from build123d import *

# Parameters (mm, degrees)
F0_W          = 40.64
F0_H          = 3.81
F1_DEPTH      = 12.7
F2_DEPTH      = 12.6492
F2_DEPTH_BACK = 12.7
F3_D          = 2.54
F3_DEPTH      = 12.701
F4_D          = 2.54
F6_DEPTH      = 4.2291
F7_DEPTH      = 4.2291
F8_D          = 3.81


with BuildPart() as f1:
    # F0 (on Front) → F1 (new body, symmetric)
    with BuildSketch(Plane.XZ):
        Rectangle(F0_W, F0_H)
    extrude(amount=F1_DEPTH, both=True)

    # F0 (on Front) → F2 (join, two sides)
    with BuildSketch(Plane.XZ) as f2_sk:
        with BuildLine():
            Line((20.32, 1.905), (20.32, -1.905))
            Line((20.32, -1.905), (29.8843930952, -0.4539235519))
            ThreePointArc((29.8843930952, -0.4539235519), (29.1094185103, 1.3335), (29.3193590481, 3.2703514481))
            Line((29.3193590481, 3.2703514481), (20.32, 1.905))
        make_face()
        with BuildLine():
            Line((32.8763121576, 0), (29.8843930952, -0.4539235519))
            ThreePointArc((29.8843930952, -0.4539235519), (34.1246887779, -1.6946744039), (36.6863121576, 1.905))
            ThreePointArc((36.6863121576, 1.905), (33.5706134801, 5.6512041687), (29.3193590481, 3.2703514481))
            Line((29.3193590481, 3.2703514481), (32.8763121576, 3.81))
            Line((32.8763121576, 3.81), (32.8763121576, 0))
        make_face()
        with BuildLine():
            ThreePointArc((29.3193590481, 3.2703514481), (29.1094185103, 1.3335), (29.8843930952, -0.4539235519))
            Line((29.8843930952, -0.4539235519), (32.8763121576, 0))
            Line((32.8763121576, 0), (32.8763121576, 3.81))
            Line((32.8763121576, 3.81), (29.3193590481, 3.2703514481))
        make_face()
        with BuildLine():
            Line((-29.8843930952, -0.4539235519), (-20.32, -1.905))
            Line((-20.32, -1.905), (-20.32, 1.905))
            Line((-20.32, 1.905), (-29.3193590481, 3.2703514481))
            ThreePointArc((-29.3193590481, 3.2703514481), (-29.1301079889, 2.5993013225), (-29.0663121576, 1.905))
            ThreePointArc((-29.0663121576, 1.905), (-29.2766377538, 0.6566233797), (-29.8843930952, -0.4539235519))
        make_face()
        with BuildLine():
            ThreePointArc((-29.3193590481, 3.2703514481), (-36.6432058049, 2.4765), (-29.8843930952, -0.4539235519))
            Line((-29.8843930952, -0.4539235519), (-32.8763121576, 0))
            Line((-32.8763121576, 0), (-32.8763121576, 3.81))
            Line((-32.8763121576, 3.81), (-29.3193590481, 3.2703514481))
        make_face()
        with BuildLine():
            Line((-32.8763121576, 0), (-29.8843930952, -0.4539235519))
            ThreePointArc((-29.8843930952, -0.4539235519), (-29.2766377538, 0.6566233797), (-29.0663121576, 1.905))
            ThreePointArc((-29.0663121576, 1.905), (-29.1301079889, 2.5993013225), (-29.3193590481, 3.2703514481))
            Line((-29.3193590481, 3.2703514481), (-32.8763121576, 3.81))
            Line((-32.8763121576, 3.81), (-32.8763121576, 0))
        make_face()
    extrude(amount=F2_DEPTH)
    extrude(f2_sk.sketch, amount=-F2_DEPTH_BACK)

    # F3 (through all, one way)
    with BuildSketch(Plane.XZ):
        with Locations((32.8763121576, 1.905), (-32.8763121576, 1.905)):
            Circle(F3_D / 2)
    extrude(amount=-F3_DEPTH, mode=Mode.SUBTRACT)

    # F4 (through all)
    with Locations(Plane(origin=(0, 0, 0), x_dir=(1, 0, 0), z_dir=(0, 1, 0))):
        with Locations((32.8763121576, -1.905), (-32.8763121576, -1.905)):
            Hole(F4_D / 2)

    # F0 (on Front) → F6 (cut, symmetric)
    with BuildSketch(Plane.XZ):
        with BuildLine():
            Line((20.32, 1.905), (20.32, -1.905))
            Line((20.32, -1.905), (29.8843930952, -0.4539235519))
            ThreePointArc((29.8843930952, -0.4539235519), (29.1094185103, 1.3335), (29.3193590481, 3.2703514481))
            Line((29.3193590481, 3.2703514481), (20.32, 1.905))
        make_face()
        with BuildLine():
            Line((32.8763121576, 0), (29.8843930952, -0.4539235519))
            ThreePointArc((29.8843930952, -0.4539235519), (34.1246887779, -1.6946744039), (36.6863121576, 1.905))
            ThreePointArc((36.6863121576, 1.905), (33.5706134801, 5.6512041687), (29.3193590481, 3.2703514481))
            Line((29.3193590481, 3.2703514481), (32.8763121576, 3.81))
            Line((32.8763121576, 3.81), (32.8763121576, 0))
        make_face()
        with BuildLine():
            ThreePointArc((29.3193590481, 3.2703514481), (29.1094185103, 1.3335), (29.8843930952, -0.4539235519))
            Line((29.8843930952, -0.4539235519), (32.8763121576, 0))
            Line((32.8763121576, 0), (32.8763121576, 3.81))
            Line((32.8763121576, 3.81), (29.3193590481, 3.2703514481))
        make_face()
    extrude(amount=F6_DEPTH, both=True, mode=Mode.SUBTRACT)

    # F0 (on Front) → F7 (cut, symmetric)
    with BuildSketch(Plane.XZ):
        with BuildLine():
            Line((-29.8843930952, -0.4539235519), (-20.32, -1.905))
            Line((-20.32, -1.905), (-20.32, 1.905))
            Line((-20.32, 1.905), (-29.3193590481, 3.2703514481))
            ThreePointArc((-29.3193590481, 3.2703514481), (-29.1301079889, 2.5993013225), (-29.0663121576, 1.905))
            ThreePointArc((-29.0663121576, 1.905), (-29.2766377538, 0.6566233797), (-29.8843930952, -0.4539235519))
        make_face()
        with BuildLine():
            Line((-32.8763121576, 0), (-29.8843930952, -0.4539235519))
            ThreePointArc((-29.8843930952, -0.4539235519), (-29.2766377538, 0.6566233797), (-29.0663121576, 1.905))
            ThreePointArc((-29.0663121576, 1.905), (-29.1301079889, 2.5993013225), (-29.3193590481, 3.2703514481))
            Line((-29.3193590481, 3.2703514481), (-32.8763121576, 3.81))
            Line((-32.8763121576, 3.81), (-32.8763121576, 0))
        make_face()
        with BuildLine():
            ThreePointArc((-29.3193590481, 3.2703514481), (-36.6432058049, 2.4765), (-29.8843930952, -0.4539235519))
            Line((-29.8843930952, -0.4539235519), (-32.8763121576, 0))
            Line((-32.8763121576, 0), (-32.8763121576, 3.81))
            Line((-32.8763121576, 3.81), (-29.3193590481, 3.2703514481))
        make_face()
    extrude(amount=F7_DEPTH, both=True, mode=Mode.SUBTRACT)

    # F8 (through all)
    with Locations(Plane.XY.offset(1.905)):
        with Locations((-15.24, 0), (15.24, 0)):
            Hole(F8_D / 2)


solid = f1.part
CAD build for the part. Positions are in the model's coordinates, mm. A direction names the side the tool comes from. Coordinates: 2 decimals unless noted, no trailing zeros. Write each loop counter-clockwise with the first axis right and the second up, starting at its lowest first coordinate (ties: lowest second). Pieces come first, ordered by that corner, then holes. Notation, with made-up numbers: M 61.25,-8 L 99.25,-8 A23 cw 99.25,21 Z; hole C 3.25,28.25 d5. An arc over 180 degrees is marked long. Answer as a JSON object with one key per item and string values. Group by question number.
1) Wall check: line 1 (X direction, y = 10.75, z = 1.75); line 2 (Y direction, x = -30.5, z = 1.5); line 3 (X direction, y = 0.5, z = 0). Give the ranges that are in metal, low to high. Write a range as from..to.
2) Saw through at A-A (x = 15.24). Write the cut outline in (y, z) (3 decimals), plus the area to 3 significant figures.
3) Saw through at D-D (z = 4.25). Write the cut outline in (x, y).
4) Saw through at B-B (y = 0). Write the cut outline in (x, z) (3 decimals).
5) Saw through at C-C (y = -11). Write the cut outline in (x, z) (3 decimals), plus the area to 3 significant figures.
6) Pin check, flat tips, straight feed: pin 1 Ø7.5 at (x, y) = (1.5, -2) entering from +Z (3 decimals); pin 2 Ø2.5 at (x, z) = (29.5, 3) entering from -Y; pin 3 Ø5 at (x, y) = (24, 7.5) entering from -Z. Stop position of each tip, or through.
7) Tool access for faces 1 (the face through (-29, -12.649, 1)), 2 (the face through (-24.76, -8.5, 2.58)), 3 (the face through (25.04, 8.41, -1.19)), 4 (the face through (28, -12.649, 1)): list every direction of +Z, -Z, +X, -X, +Y, -Y with a clear straight run to the whole face (end or side of a thin tool).
8) Mould opens along Y. For faces 5 (the face through (-36.62, -8.5, 2.61)), 6 (the face through (28, 4.229, 1)), 7 (the face through (0, -12.7, 0)), 8 (the face through (-20.32, 0, 0)) say: +Y half, -Y half, draft (parallel to the pull), parting line (faces both ways), or undercut.
Values follow:
{
 "1": {"line 1": "x = -36.68..-34.14, -31.62..31.62, 34.14..36.68", "line 2": "y = -12.65..-4.23, 4.23..12.7", "line 3": "x = -20.32..-17.08, -13.4..13.4, 17.08..20.32"},
 "2": {"outline": "M -12.7,-1.905 L -1.905,-1.905 L -1.905,1.905 L -12.7,1.905 Z; M 1.905,-1.905 L 12.7,-1.905 L 12.7,1.905 L 1.905,1.905 Z", "area": "82.3 mm2"},
 "3": {"outline": "M -35.88,-12.65 L -29.87,-12.65 L -29.87,-4.23 L -35.88,-4.23 Z; M -35.88,4.23 L -29.87,4.23 L -29.87,12.7 L -35.88,12.7 Z; M 29.87,-12.65 L 35.88,-12.65 L 35.88,-4.23 L 29.87,-4.23 Z; M 29.87,4.23 L 35.88,4.23 L 35.88,12.7 L 29.87,12.7 Z"},
 "4": {"outline": "M -20.32,-1.905 L -17.145,-1.905 L -17.145,1.905 L -20.32,1.905 Z; M -13.335,-1.905 L 13.335,-1.905 L 13.335,1.905 L -13.335,1.905 Z; M 17.145,-1.905 L 20.32,-1.905 L 20.32,1.905 L 17.145,1.905 Z"},
 "5": {"outline": "M -29.884,-0.454 L -20.32,-1.905 L 20.32,-1.905 L 29.884,-0.454 A3.81 ccw long 29.319,3.27 L 20.32,1.905 L -20.32,1.905 L -29.319,3.27 A3.81 ccw long Z; hole C -32.876,1.905 d2.54; hole C 32.876,1.905 d2.54", "area": "304 mm2"},
 "6": {"pin 1": "stops at z = 1.905", "pin 2": "stops at y = -12.65", "pin 3": "stops at z = -1.73"},
 "7": {"face 1": "+Z, -Z, -X, -Y", "face 2": "+Z, +Y, -Y", "face 3": "-Z, +Y, -Y", "face 4": "+Z, -Z, +X, -Y"},
 "8": {"face 5": "draft", "face 6": "undercut", "face 7": "-Y half", "face 8": "undercut"}
}
